Can you work these out from the drawing? Everything is in mm from the part's minimum corner. A direction names the side the tool comes from. Round coordinates to 2 decimals unless told otherwise and drop trailing zeros. Write each loop counter-clockwise with the first axis right and the second up, starting at its lowest first coordinate (ties: lowest second). Pieces come first, ordered by that corner, then holes.
Q1. If we section it at D-D (z = 20): Please give me the cut outline in (x, y).
Q2. If we section it at B-B (x = 18): Please give me the cut outline in (y, z).
Q3. I'm going to push flat-ended pins straight in: pin 1 Ø0.6 at (y, z) = (45.5, 21) entering from -X; pin 2 Ø10.5 at (x, z) = (15.5, 9.5) entering from -Y; pin 3 Ø2 at (y, z) = (18.5, 18) entering from +X. Where does each tip first touch, or does it pass through?
Q4. For the marked faces 1, 2, 3, 4 and 5, which set-ups out of +Z, -Z, +X, -X, +Y, -Y let a thin tool reach every point of the face, with its end or its side?
Q5. If we section it at A-A (z = 27): Please give me the cut outline in (x, y) (1 decimal), plus the area to 3 significant figures.
Q6. Please list where these lines run through material, in increasing order: line 1 along Y through (x, z) = (13, 14.5); line 2 along Y through (x, z) = (7.25, 19.5); line 3 along Y through (x, z) = (1.5, 19.5).
Q7. If we section it at C-C (y = 45): Please give me the cut outline in (x, z).
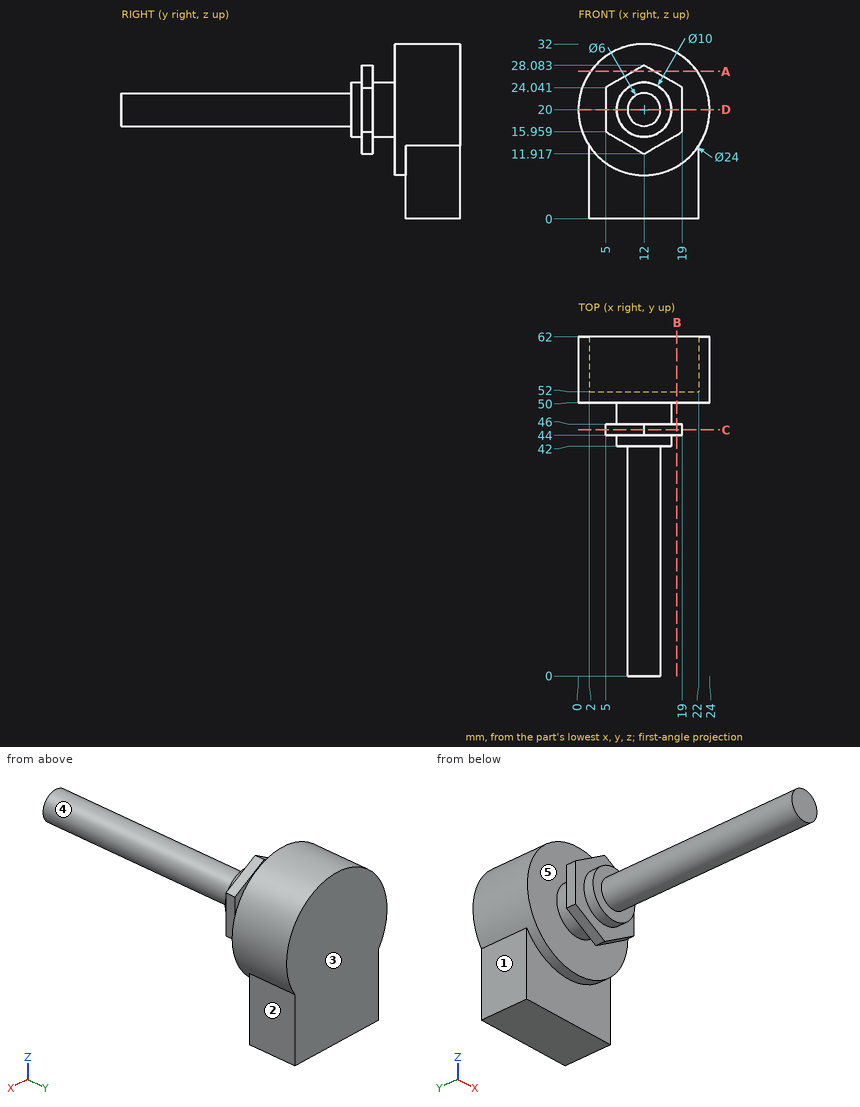
A:
1. outline: (0, 50) - (7, 50) - (7, 46) - (5, 46) - (5, 44) - (7, 44) - (7, 42) - (9, 42) - (9, 0) - (15, 0) - (15, 42) - (17, 42) - (17, 44) - (19, 44) - (19, 46) - (17, 46) - (17, 50) - (24, 50) - (24, 62) - (0, 62) - close
2. outline: (44, 15.38) - (46, 15.38) - (46, 24.62) - (44, 24.62) - close; (50, 9.61) - (52, 9.61) - (52, 0) - (62, 0) - (62, 30.39) - (50, 30.39) - close
3. pin 1: stops at x = 5
3. pin 2: stops at y = 44
3. pin 3: stops at x = 14.83
4. face 1: -Z, -X, +Y, -Y
4. face 2: -Z, +X, +Y, -Y
4. face 3: +Z, -Z, +X, -X, +Y
4. face 4: -Y
4. face 5: none
5. outline: (2.3, 50) - (21.7, 50) - (21.7, 62) - (2.3, 62) - close; (10.1, 44) - (13.9, 44) - (13.9, 46) - (10.1, 46) - close
5. area: 241 mm2
6. line 1: y = 44 to 46, 50 to 62
6. line 2: y = 42 to 62
6. line 3: y = 50 to 62
7. outline: (5, 15.96) - (12, 11.92) - (19, 15.96) - (19, 24.04) - (12, 28.08) - (5, 24.04) - close
